from build123d import *

# Parameters (mm, degrees)
EXTRUDE_3_DEPTH = 400


with BuildPart() as part:
    # 草图30 → 凸台-拉伸3 (new body)
    with BuildSketch(Plane.XY):
        with BuildLine():
            Line((0.8, 4.385786438), (4.664213562, 8.25))
            Line((4.664213562, 8.25), (8, 8.25))
            Line((8, 8.25), (8, 4.1))
            Line((8, 4.1), (9.2, 4.1))
            Line((9.2, 4.1), (9.2, 5.1))
            Line((9.2, 5.1), (10, 5.1))
            Line((10, 5.1), (10, 19))
            ThreePointArc((10, 19), (9.707106781, 19.707106781), (9, 20))
            Line((9, 20), (4.878384215, 20))
            Line((4.878384215, 20), (4.878384215, 19.2))
            Line((4.878384215, 19.2), (3.878384215, 19.2))
            Line((3.878384215, 19.2), (3.878384215, 18))
            Line((3.878384215, 18), (8.028384215, 18))
            Line((8.028384215, 18), (8.028384215, 14.664213562))
            Line((8.028384215, 14.664213562), (4.164170652, 10.8))
            Line((4.164170652, 10.8), (-4.607402223, 10.8))
            Line((-4.607402223, 10.8), (-8.471615785, 14.664213562))
            Line((-8.471615785, 14.664213562), (-8.471615785, 18))
            Line((-8.471615785, 18), (-4.321615785, 18))
            Line((-4.321615785, 18), (-4.321615785, 19.2))
            Line((-4.321615785, 19.2), (-5.321615785, 19.2))
            Line((-5.321615785, 19.2), (-5.321615785, 20))
            Line((-5.321615785, 20), (-9, 20))
            ThreePointArc((-9, 20), (-9.707106781, 19.707106781), (-10, 19))
            Line((-10, 19), (-10, -19))
            ThreePointArc((-10, -19), (-9.707106781, -19.707106781), (-9, -20))
            Line((-9, -20), (-5.321615785, -20))
            Line((-5.321615785, -20), (-5.321615785, -19.2))
            Line((-5.321615785, -19.2), (-4.321615785, -19.2))
            Line((-4.321615785, -19.2), (-4.321615785, -18))
            Line((-4.321615785, -18), (-8.471615785, -18))
            Line((-8.471615785, -18), (-8.471615785, -14.664213562))
            Line((-8.471615785, -14.664213562), (-4.607402223, -10.8))
            Line((-4.607402223, -10.8), (4.164170652, -10.8))
            Line((4.164170652, -10.8), (8.028384215, -14.664213562))
            Line((8.028384215, -14.664213562), (8.028384215, -18))
            Line((8.028384215, -18), (3.878384215, -18))
            Line((3.878384215, -18), (3.878384215, -19.2))
            Line((3.878384215, -19.2), (4.878384215, -19.2))
            Line((4.878384215, -19.2), (4.878384215, -20))
            Line((4.878384215, -20), (9, -20))
            ThreePointArc((9, -20), (9.707106781, -19.707106781), (10, -19))
            Line((10, -19), (10, -5.1))
            Line((10, -5.1), (9.2, -5.1))
            Line((9.2, -5.1), (9.2, -4.1))
            Line((9.2, -4.1), (8, -4.1))
            Line((8, -4.1), (8, -8.25))
            Line((8, -8.25), (4.664213562, -8.25))
            Line((4.664213562, -8.25), (0.8, -4.385786438))
            Line((0.8, -4.385786438), (0.8, 4.385786438))
        make_face()
        with BuildLine():
            Line((-1.7, 7.3), (-1.7, -7.3))
            ThreePointArc((-1.7, -7.3), (-1.992893219, -8.007106781), (-2.7, -8.3))
            Line((-2.7, -8.3), (-6.5, -8.3))
            ThreePointArc((-6.5, -8.3), (-7.207106781, -8.007106781), (-7.5, -7.3))
            Line((-7.5, -7.3), (-7.5, 7.3))
            ThreePointArc((-7.5, 7.3), (-7.207106781, 8.007106781), (-6.5, 8.3))
            Line((-6.5, 8.3), (-2.7, 8.3))
            ThreePointArc((-2.7, 8.3), (-1.992893219, 8.007106781), (-1.7, 7.3))
        make_face(mode=Mode.SUBTRACT)
    extrude(amount=EXTRUDE_3_DEPTH)


solid = part.part
Source: CAD feature listing. Evaluate the final solid. Frame: model axes, mm. A direction names the side the tool comes from. Round coordinates to 2 decimals unless told otherwise and drop trailing zeros. Loops run counter-clockwise (first coordinate to the right, second up) from the corner with the lowest first, then second, coordinate; pieces in that order, holes last. Notation, with made-up numbers: (-30, -19) - (-4, -19) arc R27 cw to (-4, 17) - close; hole circle Ø8 at (-23.5, 87.5). An arc over 180 degrees is marked (long way). Write item = value, one per line. Start each with the question number.
(1) Pin query (flat end, axial travel): pin 1 (2.5 mm diameter, centred on x = 1, z = 278, fed in from -Y); pin 2 (4 mm diameter, centred on x = 2, z = 244, fed in from -Y); pin 3 (0.6 mm diameter, centred on y = -19.5, z = 210, fed in from -X); pin 4 (5 mm diameter, centred on x = -1, y = -10, fed in from -Z). Return the tip coordinate at first contact, or that it passes through.
(2) Section query A-A, the plane y = 0. Output: boundary loops of the cut face in (x, z), plus the area to 3 significant figures.
(3) Pull-direction query (Y, two-part tool) for faces 3 (the face through (0, 0, 0)), 4 (the face through (-7.5, 0, 197)); classes: +Y half, -Y half, draft (parallel to the pull), parting line (faces both ways), or undercut.
(4) Set-up query: faces 1 (the face through (-1.7, 0, 197)), 2 (the face through (10, -12, 197)). Return all of +Z, -Z, +X, -X, +Y, -Y with unobstructed straight access to the full face (end or side cutting, diameter ignored); none if empty.
(5) Ray query, line 1 along X through (y, z) = (-8, 373); line 2 along Y through (x, z) = (5, 92); line 3 along Y through (x, z) = (6.75, 52.5). Return the intervals inside material, ascending. Write a range as from..to.
Conclusion:
q1.pin_1 = -10.8
q1.pin_2 = -19.2
q1.pin_3 = -9.98
q1.pin_4 = 0
q2.outline = (-10, 0) - (-7.5, 0) - (-7.5, 400) - (-10, 400) - close; (-1.7, 0) - (0.8, 0) - (0.8, 400) - (-1.7, 400) - close
q2.area = 2,000 mm2
q3.face_3 = draft
q3.face_4 = undercut
q4.face_1 = +Z, -Z
q4.face_2 = +Z, -Z, +X, +Y, -Y
q5.line_1 = -10..-7.21, -1.99..4.41, 8..10
q5.line_2 = -20..-18, -11.64..-8.25, 8.25..11.64, 18..20
q5.line_3 = -20..-18, -13.39..-8.25, 8.25..13.39, 18..20
